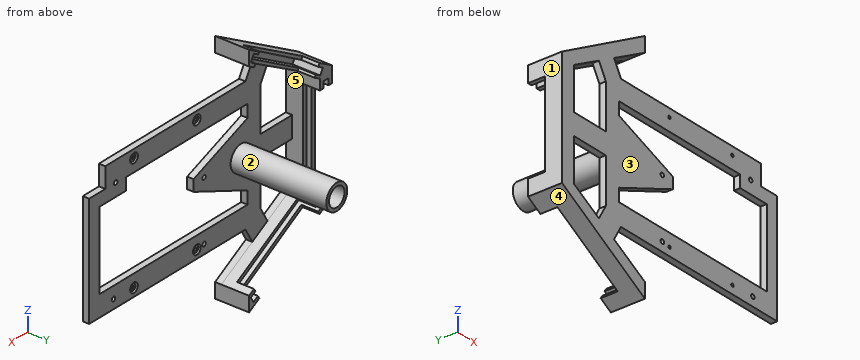
```python
from build123d import *

# Parameters (mm, degrees)
BOSS_EXTRUDE1_DEPTH                         = 3
BOSS_EXTRUDE7_DEPTH                         = 13
SKETCH14_W                                  = 3
SKETCH14_H                                  = 46
CUT_EXTRUDE1_DEPTH                          = 13
SKETCH15_W                                  = 7
SKETCH15_H                                  = 40
CUT_EXTRUDE3_DEPTH                          = 8
CUT_EXTRUDE5_REACH                          = 97.01
SKETCH18_R                                  = 6
SKETCH18_R_2                                = 4.445
BOSS_EXTRUDE8_DEPTH                         = 45
CBORE_FOR_00_BINDING_HEAD_MACHINE_S_2_COUNT = 2
CBORE_FOR_00_BINDING_HEAD_MACHINE_S_2_PITCH = 54.28
CBORE_FOR_00_BINDING_HEAD_MACHINE_S_3_COUNT = 2
CBORE_FOR_00_BINDING_HEAD_MACHINE_S_3_PITCH = 65.199484661
CBORE_FOR_00_BINDING_HEAD_MACHINE_S_4_COUNT = 2
CBORE_FOR_00_BINDING_HEAD_MACHINE_S_4_PITCH = 36.12
SKETCH22_R                                  = 1
CUT_EXTRUDE6_DEPTH                          = 105.321261807
CUT_EXTRUDE8_DEPTH                          = 105.321261807
SKETCH24_W                                  = 9.24
SKETCH24_H                                  = 9.529738598
CUT_EXTRUDE9_DEPTH                          = 105.321261807


with BuildPart() as part:
    # Sketch1 → Boss-Extrude1 (new body)
    with BuildSketch(Plane(origin=(0, 0, 0), x_dir=(1, 0, 0), z_dir=(0, 1, 0))):
        Polygon((-76.37359272, 27.5), (-76.37359272, -27.5), (-28.742195512, -55), (-28.742195512, -31), (47.257804488, -31), (47.257804488, 31), (-28.742195512, 31), (-28.742195512, 55), align=None)
    extrude(amount=BOSS_EXTRUDE1_DEPTH)

    # Sketch11 → Boss-Extrude7 (add)
    with BuildSketch(Plane(origin=(0, 3, 0), x_dir=(1, 0, 0), z_dir=(0, 1, 0))):
        Polygon((-28.742195512, -55), (-28.742195512, -48), (-69.37359272, -24.979495292), (-69.37359272, 24.979495292), (-28.742195512, 48), (-28.742195512, 55), (-76.37359272, 27.5), (-76.37359272, -27.5), align=None)
    extrude(amount=BOSS_EXTRUDE7_DEPTH)

    # Sketch14 → Cut-Extrude1 (cut)
    with BuildSketch(Plane(origin=(0, 16, 0), x_dir=(1, 0, 0), z_dir=(0, 1, 0))):
        Polygon((-29.742195512, 49.210281508), (-69.579364086, 26.210281508), (-71.079364086, 28.80835772), (-31.242195512, 51.80835772), align=None)
        with Locations((-72.87359272, 0)):
            Rectangle(SKETCH14_W, SKETCH14_H)
        Polygon((-71.079364086, -28.80835772), (-31.476965636, -52.210281508), (-29.742195512, -49.210281508), (-69.579364086, -26.210281508), align=None)
    extrude(amount=-CUT_EXTRUDE1_DEPTH, mode=Mode.SUBTRACT)

    # Sketch15 → Cut-Extrude3 (cut)
    with BuildSketch(Plane(origin=(0, 16, 0), x_dir=(1, 0, 0), z_dir=(0, 1, 0))):
        with Locations((-72.87359272, 0)):
            Rectangle(SKETCH15_W, SKETCH15_H)
        Polygon((-69.238309522, 31.619557675), (-66.423300051, 26.651040721), (-31.579449527, 46.392498809), (-34.59729337, 51.619557675), align=None)
        Polygon((-66.396023158, -26.666494973), (-69.251333812, -31.612038098), (-34.568999008, -51.635893433), (-31.593683239, -46.384434424), align=None)
    extrude(amount=-CUT_EXTRUDE3_DEPTH, mode=Mode.SUBTRACT)

    # Sketch17 → Cut-Extrude5 (cut, up to next)
    with BuildSketch(Plane(origin=(0, 3, 0), x_dir=(1, 0, 0), z_dir=(0, 1, 0)), mode=Mode.PRIVATE) as cut_extrude5_sk1:
        Polygon((-69.37359272, -24.979495292), (-69.37359272, -5.130907192), (-51.219056623, -5.130907192), (-51.219056623, -26.070515137), (-55.162644513, -33.030983121), align=None)
    cut_extrude5_tool1 = extrude(cut_extrude5_sk1.sketch, amount=-CUT_EXTRUDE5_REACH, mode=Mode.PRIVATE) & part.part
    # Sketch17 → Cut-Extrude5 (cut, up to next)
    with BuildSketch(Plane(origin=(0, 3, 0), x_dir=(1, 0, 0), z_dir=(0, 1, 0)), mode=Mode.PRIVATE) as cut_extrude5_sk2:
        Polygon((-69.37359272, 24.979495292), (-69.37359272, 4.869092808), (-51.219056623, 4.869092808), (-51.219056623, 26.070515137), (-55.162644513, 33.030983121), align=None)
    cut_extrude5_tool2 = extrude(cut_extrude5_sk2.sketch, amount=-CUT_EXTRUDE5_REACH, mode=Mode.PRIVATE) & part.part
    # Sketch17 → Cut-Extrude5 (cut, up to next)
    with BuildSketch(Plane(origin=(0, 3, 0), x_dir=(1, 0, 0), z_dir=(0, 1, 0)), mode=Mode.PRIVATE) as cut_extrude5_sk3:
        Polygon((-28.742195512, -48), (-46.462059534, -37.960467984), (-42.518471644, -31), (-28.742195512, -31), align=None)
    cut_extrude5_tool3 = extrude(cut_extrude5_sk3.sketch, amount=-CUT_EXTRUDE5_REACH, mode=Mode.PRIVATE) & part.part
    # Sketch17 → Cut-Extrude5 (cut, up to next)
    with BuildSketch(Plane(origin=(0, 3, 0), x_dir=(1, 0, 0), z_dir=(0, 1, 0)), mode=Mode.PRIVATE) as cut_extrude5_sk4:
        Polygon((-28.742195512, 31), (-42.518471644, 31), (-46.462059534, 37.960467984), (-28.742195512, 48), align=None)
    cut_extrude5_tool4 = extrude(cut_extrude5_sk4.sketch, amount=-CUT_EXTRUDE5_REACH, mode=Mode.PRIVATE) & part.part
    add(cut_extrude5_tool1.solids().sort_by_distance((-59.97086, 3, 17.234777))[0], mode=Mode.SUBTRACT)
    add(cut_extrude5_tool2.solids().sort_by_distance((-59.974373, 3, -17.10271))[0], mode=Mode.SUBTRACT)
    add(cut_extrude5_tool3.solids().sort_by_distance((-35.757612, 3, 37.618563))[0], mode=Mode.SUBTRACT)
    add(cut_extrude5_tool4.solids().sort_by_distance((-35.757612, 3, -37.618563))[0], mode=Mode.SUBTRACT)

    # Sketch18 → Boss-Extrude8 (add)
    with BuildSketch(Plane(origin=(0, 3, 0), x_dir=(1, 0, 0), z_dir=(0, 1, 0))):
        with Locations(Location((-40, 0, 0), (0, 0, 90))):
            Circle(SKETCH18_R)
        with Locations(Location((-40, 0, 0), (0, 0, 90))):
            Circle(SKETCH18_R_2, mode=Mode.SUBTRACT)
    extrude(amount=BOSS_EXTRUDE8_DEPTH)

    # Sketch21 → CBORE for #00 Binding Head Machine Screw1 (revolve, cut)
    with BuildSketch(Plane(origin=(-14.622195512, 3, 27.14), x_dir=(0, 0, 1), z_dir=(1, 0, 0))):
        Polygon((0, 0), (0, 3), (0.6985, 3), (0.6985, 0.7112), (1.5875, 0.7112), (1.5875, 0.635), (2.2225, 0), align=None)
    cbore_for_00_binding_head_machine_screw = revolve(axis=Axis((-14.622195512, 9.35, 27.14), (0, -1, 0)), mode=Mode.SUBTRACT)

    # CBORE for _00 Binding Head Machine S 2: CBORE for #00 Binding Head Machine Screw1 ×2
    with Locations(*[(0, 0, -i * CBORE_FOR_00_BINDING_HEAD_MACHINE_S_2_PITCH) for i in range(1, CBORE_FOR_00_BINDING_HEAD_MACHINE_S_2_COUNT)]):
        add(cbore_for_00_binding_head_machine_screw, mode=Mode.SUBTRACT)

    # CBORE for _00 Binding Head Machine S 3: CBORE for #00 Binding Head Machine Screw1 ×2
    with Locations(*[Vector(0.5539921088035915, 0, -0.832521917659439) * (i * CBORE_FOR_00_BINDING_HEAD_MACHINE_S_3_PITCH) for i in range(1, CBORE_FOR_00_BINDING_HEAD_MACHINE_S_3_COUNT)]):
        add(cbore_for_00_binding_head_machine_screw, mode=Mode.SUBTRACT)

    # CBORE for _00 Binding Head Machine S 4: CBORE for #00 Binding Head Machine Screw1 ×2
    with Locations(*[(i * CBORE_FOR_00_BINDING_HEAD_MACHINE_S_4_PITCH, 0, 0) for i in range(1, CBORE_FOR_00_BINDING_HEAD_MACHINE_S_4_COUNT)]):
        add(cbore_for_00_binding_head_machine_screw, mode=Mode.SUBTRACT)

    # Sketch22 → Cut-Extrude6 (cut, through all)
    with BuildSketch(Plane(origin=(0, 3, 0), x_dir=(1, 0, 0), z_dir=(0, 1, 0))):
        with Locations(Location((33.287804488, 26.734999831, 0), (0, 0, 270))):
            Circle(SKETCH22_R)
        with Locations(Location((32.017804488, -21.470261402, 0), (0, 0, 270))):
            Circle(SKETCH22_R)
        with Locations(Location((-18.742195512, 26.67, 0), (0, 0, 270))):
            Circle(SKETCH22_R)
        with Locations(Location((-18.742195512, -1.26, 0), (0, 0, 270))):
            Circle(SKETCH22_R)
    extrude(amount=-CUT_EXTRUDE6_DEPTH, mode=Mode.SUBTRACT)

    # Sketch23 → Cut-Extrude8 (cut, through all)
    with BuildSketch(Plane(origin=(0, 3, 0), x_dir=(1, 0, 0), z_dir=(0, 1, 0))):
        Polygon((-43.742195512, 21.14), (-43.742195512, 15.14), (-12.742195512, 2.140015237), (-12.742195512, -3.206984729), (-43.742195512, -15.14), (-43.742195512, -21.14), (26.017804488, -21.14), (26.017804488, -15.470261402), (41.257804488, -15.470261402), (41.257804488, 21.14), align=None)
    extrude(amount=-CUT_EXTRUDE8_DEPTH, mode=Mode.SUBTRACT)

    # Sketch24 → Cut-Extrude9 (cut, through all)
    with BuildSketch(Plane(origin=(0, 3, 0), x_dir=(1, 0, 0), z_dir=(0, 1, 0))):
        with Locations((42.637804488, -26.235130701)):
            Rectangle(SKETCH24_W, SKETCH24_H)
    extrude(amount=-CUT_EXTRUDE9_DEPTH, mode=Mode.SUBTRACT)


solid = part.part
```
CAD build for the part. Positions are in the model's coordinates, mm. Face numbers are marked on the shaded views. A direction names the side the tool comes from. Round coordinates to 2 decimals unless told otherwise and drop trailing zeros. Write each loop counter-clockwise with the first axis right and the second up, starting at its lowest first coordinate (ties: lowest second). Pieces come first, ordered by that corner, then holes. Notation, with made-up numbers: (45, 47.5) - (91, 47.5) arc R12 cw to (91, 69.5) - close; hole circle Ø9 at (34.25, 27). An arc over 180 degrees is marked (long way). Write item = value, one per line. Start each with the question number.
Q1. Drop flat-ended pins along their axis: pin 1 (2.5 mm diameter, centred on x = 0, y = 2, fed in from -Z); pin 2 (10 mm diameter, centred on x = -28, y = 29, fed in from -Z); pin 3 (1.6 mm diameter, centred on x = -70.5, z = -1.5, fed in from +Y); pin 4 (2 mm diameter, centred on x = -75.5, y = 13, fed in from +Z). Give the stop position or say it passes through.
Q2. Which spindle directions (+Z, -Z, +X, -X, +Y, -Y) get a long thin tool onto all of the face, cutting with end or side? Do the marked faces 1 and 2. Say none if no direction does.
Q3. Band-saw the part on B-B (x = 13). Give the cut face in (y, z).
Q4. Mould opens along Z. For the marked faces 3, 4 and 5 say: pulls with the +Z half, pulls with the -Z half, needs draft (parallel to the pull), parting line crosses it, or undercut.
Q5. Band-saw the part on C-C (x = -65). Give the cut face in (y, z).
Q6. Band-saw the part on D-D (y = 39.5). Give the cut face in (x, z) (3 decimals), then the cut area to 3 significant figures.
Q7. Probe L1, parallel to Z at x = -40, y = 39.5 (3 decimals); L2, parallel to X at y = 1, z = -27; L3, parallel to X at y = 2.35, z = -27.14 (3 decimals). List the from-to ranges inside material, lowest first. Write a range as from..to.
Q8. Band-saw the part on A-A (y = 5.5). Give the cut face in (x, z) (1 decimal).
Answers below:
q1.pin_1 = -31
q1.pin_2 = through
q1.pin_3 = 8
q1.pin_4 = 28.58
q2.face_1 = +Z, -Z, -X, +Y, -Y
q2.face_2 = +Y
q3.outline = (0, -31) - (3, -31) - (3, -21.14) - (0, -21.14) - close; (0, 21.14) - (3, 21.14) - (3, 31) - (0, 31) - close
q4.face_3 = needs draft
q4.face_4 = pulls with the -Z half
q4.face_5 = undercut
q5.outline = (0, -34.07) - (8, -34.07) - (8, -32.32) - (3, -32.32) - (3, -28.85) - (8, -28.85) - (8, -27.46) - (0, -27.46) - close; (0, -4.87) - (3, -4.87) - (3, 5.13) - (0, 5.13) - close; (0, 27.46) - (8, 27.46) - (8, 28.85) - (3, 28.85) - (3, 32.4) - (8, 32.4) - (8, 34.07) - (0, 34.07) - close
q6.outline = circle Ø12 at (-40, 0); hole circle Ø8.89 at (-40, 0)
q6.area = 51.0 mm2
q7.L1 = -6..-4.445, 4.445..6
q7.L2 = -76.37..-65.81, -51.75..-19.69, -17.8..-15.31, -13.94..20.81, 22.18..32.32, 34.25..47.26
q7.L3 = -76.374..-65.56, -51.825..-19.625, -17.86..-16.21, -13.035..19.91, 23.085..32.373, 34.202..47.258
q8.outline = (-76.4, -27.5) - (-28.7, -55) - (-28.7, -48) - (-69.4, -25) - (-69.4, 25) - (-28.7, 48) - (-28.7, 55) - (-76.4, 27.5) - close; circle Ø12 at (-40, 0); hole (-74.4, -23) - (-71.4, -23) - (-71.4, 23) - (-74.4, 23) - close; hole (-71.1, -28.8) - (-31.2, -51.8) - (-29.7, -49.2) - (-69.6, -26.2) - close; hole (-71.1, 28.8) - (-69.6, 26.2) - (-29.7, 49.2) - (-31.5, 52.2) - close; hole circle Ø8.9 at (-40, 0)
